```python
from build123d import *

# Parameters (mm, degrees)
BOSS_EXTRUDE1_DEPTH = 6.35
SKETCH2_R           = 3.175
SKETCH2_R_2         = 1.75
CUT_EXTRUDE1_DEPTH  = 7.35
BOSS_EXTRUDE2_DEPTH = 6.35
FILLET1_R           = 12.7
FILLET2_R           = 25.4


with BuildPart() as part:
    # Sketch1 → Boss-Extrude1 (new body)
    with BuildSketch(Plane.XY):
        with BuildLine():
            Line((-8.595455009, 68.571709933), (30.25643609, 34.276325287))
            ThreePointArc((30.25643609, 34.276325287), (37.667757847, 25.912514713), (42.82871051, 16.000623615))
            ThreePointArc((42.82871051, 16.000623615), (40.96564892, 11.91525319), (36.880278494, 13.77831478))
            ThreePointArc((36.880278494, 13.77831478), (24.419435892, 30.881840145), (4.903675305, 39.063421106))
            ThreePointArc((4.903675305, 39.063421106), (-10.270602503, 43.44261231), (-23.366607565, 52.270447493))
            ThreePointArc((-23.366607565, 52.270447493), (-24.02632087, 67.711201194), (-8.595455009, 68.571709933))
        make_face()
    extrude(amount=BOSS_EXTRUDE1_DEPTH)

    # Sketch2 → Cut-Extrude1 (cut, through all)
    with BuildSketch(Plane.XY.offset(6.35)):
        with Locations((-15.875, 60.325)):
            Circle(SKETCH2_R)
        with Locations((-10.580785461, 66.322607224)):
            Circle(SKETCH2_R_2)
        with Locations((-9.877392776, 55.030785461)):
            Circle(SKETCH2_R_2)
        with Locations((-21.169214539, 54.327392776)):
            Circle(SKETCH2_R_2)
        with Locations((-21.872607224, 65.619214539)):
            Circle(SKETCH2_R_2)
    extrude(amount=-CUT_EXTRUDE1_DEPTH, mode=Mode.SUBTRACT)

    # Sketch3 → Boss-Extrude2 (add, through all)
    with BuildSketch(Plane(origin=(0, 0, 0), x_dir=(-1, 0, 0), z_dir=(0, 0, -1))):
        with BuildLine():
            Line((-0.746918011, 60.325), (-45.72, 60.325))
            Line((-45.72, 60.325), (-45.72, 0))
            ThreePointArc((-45.72, 0), (-41.67518841, 18.801517784), (-30.25643609, 34.276325287))
            Line((-30.25643609, 34.276325287), (-0.746918011, 60.325))
        make_face()
    extrude(amount=-BOSS_EXTRUDE2_DEPTH)

    # Fillet1
    fillet1_edges = [part.edges().sort_by_distance(p)[0] for p in [
        (0.746918011, 60.325, 3.175),
    ]]
    fillet(fillet1_edges, radius=FILLET1_R)

    # Fillet2
    fillet2_edges = [part.edges().sort_by_distance(p)[0] for p in [
        (45.72, 60.325, 3.175),
    ]]
    fillet(fillet2_edges, radius=FILLET2_R)


solid = part.part
```
Geometry: final body of the model. Coordinates: model frame, mm. A direction names the side the tool comes from. Give positions to 0.01 mm unless a question says otherwise; leave off trailing zeros. Write each loop counter-clockwise with the first axis right and the second up, starting at its lowest first coordinate (ties: lowest second). Pieces come first, ordered by that corner, then holes.
1. Section query D-D, the plane y = 25.5. Return loops of the section in (x, z).
2. Section query B-B, the plane z = 1.75. Count the separate pieces of the cut face and the enclosed holes in it, then the cut area to 3 significant figures.
3. Section query A-A, the plane y = 62. Return loops of the section in (x, z).
4. Pin query (flat end, axial travel): P1, Ø1, axis at y = 42, z = 5, coming from the +X side; P2, Ø4, axis at x = -15.875, y = 60.325, coming from the -Z side; P3, Ø1.5, axis at y = 53.5, z = 4, coming from the -X side; P4, Ø1.9, axis at x = 11.5, z = 2.5, coming from the +Y side (3 decimals). Return the tip coordinate at first contact, or that it passes through.
5. Line query: probe 1 along Y at (x, z) = (-20.5, 4.75); probe 2 along X at (y, z) = (65, 2); probe 3 along Y at (x, z) = (-9.5, 6.25). Output: solid intervals per line, ascending.
6. Draft query along Y for faces 3 (the cylindrical face through (-10.96, 64.614, 3.219)), 4 (the flat face through (-5.765, 66.073, 3.131)), 5 (the cylindrical face through (24.654, 30.695, 3.131)), 6 (the cylindrical face through (-22.558, 53.263, 3.219)). Return one class per face: released by +Y, released by -Y, zero draft, split by the parting line, or undercut.
7. Section query C-C, the plane x = -17. Return loops of the section in (y, z), then the cut area to 3 significant figures.
8. Reachability of faces 1 (the flat face through (13, 60.325, 3)), 2 (the flat face through (10, 44, 6.35)) from +Z, -Z, +X, -X, +Y, -Y: full face, straight path, thin tool, end or side. Return the list, or none.
Computed:
1. outline: (30, 0) - (45.72, 0) - (45.72, 6.35) - (30, 6.35) - close
2. separate pieces: 1
2. enclosed holes: 5
2. area: 1,840 mm2
3. outline: (-26.75, 0) - (-18.57, 0) - (-18.57, 6.35) - (-26.75, 6.35) - close; (-13.18, 0) - (-0.75, 0) - (-0.75, 6.35) - (-13.18, 6.35) - close
4. P1: stops at x = 44.85
4. P2: passes through
4. P3: stops at x = -25.05
4. P4: stops at y = 60.325
5. probe 1: y = 49.8 to 52.71, 55.94 to 64.53, 66.7 to 70.31
5. probe 2: x = -25.83 to -23.51, -20.24 to -11.73, -9.43 to -4.55
5. probe 3: y = 43.09 to 53.32, 56.74 to 64.95, 67.7 to 69.29
6. face 3: undercut
6. face 4: released by +Y
6. face 5: released by -Y
6. face 6: undercut
7. outline: (47.23, 0) - (57.36, 0) - (57.36, 6.35) - (47.23, 6.35) - close; (63.29, 0) - (71.27, 0) - (71.27, 6.35) - (63.29, 6.35) - close
7. area: 115 mm2
8. face 1: +Z, -Z, +X, +Y
8. face 2: +Z, +X, -X, +Y, -Y
